Read the model definition and answer for the solid it produces. Units are mm, in the model's axes. A direction names the side the tool comes from. Coordinates: 2 decimals unless noted, no trailing zeros. Write each loop counter-clockwise with the first axis right and the second up, starting at its lowest first coordinate (ties: lowest second). Pieces come first, ordered by that corner, then holes. Notation, with made-up numbers: (-14, -2) -> (26, -2) arc R20 ccw to (26, 16) -> close; hole circle Ø7 at (18.5, 17.5). An arc over 180 degrees is marked (long way). Answer as a JSON object with one key per item and string values. Group by question number.
(1) Which of the six approach directions +Z, -Z, +X, -X, +Y, -Y give full straight-line access (tool end or side, diameter ignored) to faces 1 (the face through (-1.3, -0.6, 3)), 2 (the face through (1.2, -1.2, 0)), 3 (the face through (0, -1.25, 2))?
(2) For a pull along X with two mould halves and no side action, classify faces 4 (the face through (0, 1.25, 2)), 5 (the face through (-0.596, -2.685, 1.479)), 6 (the face through (0, 0, -11.5)) as +X half, -X half, draft (parallel to the pull), parting line (faces both ways), or undercut.
(3) Straight lines are drawn through the part: L1, parallel to Z at x = 0.4, y = 2; L2, parallel to Y at x = 2.45, z = 1.25; L3, parallel to Y at x = -0.9, z = 2. For each, find the intervals that lie inside material, in ascending order.
(4) Find section C-C (z = -0.25). Give the vertices of the cut face in (x, y), then the cut area to 3 significant figures.
(5) Flat-ended cylindrical pins translate along their axes: P1, Ø0.8, axis at x = 0, y = 0, coming from the +Z side; P2, Ø3, axis at x = -1, z = -6.5, coming from the +Y side. Find the tip coordinate at first contact, or state that the pin passes through.
(6) Find section D-D (x = 1.65). Give the vertices of the cut face in (y, z), then the cut area to 3 significant figures.
(7) Find section A-A (y = -0.7). Give the vertices of the cut face in (x, z), then the cut area to 3 significant figures.
(8) Find section B-B (x = 0). Give the vertices of the cut face in (y, z), then the cut area to 4 significant figures.
from build123d import *

# Parameters (mm, degrees)
SKETCH2_R           = 2.75
BOSS_EXTRUDE1_DEPTH = 3
SKETCH3_R           = 1.5
BOSS_EXTRUDE2_DEPTH = 11.5
CUT_EXTRUDE1_DEPTH  = 1.5


with BuildPart() as part:
    # Sketch2 → Boss-Extrude1 (new body)
    with BuildSketch(Plane.XY):
        Circle(SKETCH2_R)
    extrude(amount=BOSS_EXTRUDE1_DEPTH)

    # Sketch3 → Boss-Extrude2 (add)
    with BuildSketch(Plane(origin=(0, 0, 0), x_dir=(-1, 0, 0), z_dir=(0, 0, -1))):
        Circle(SKETCH3_R)
    extrude(amount=BOSS_EXTRUDE2_DEPTH)

    # Sketch4 → Cut-Extrude1 (cut)
    with BuildSketch(Plane.XY.offset(3)):
        Polygon((1.443375673, 0), (0.721687836, 1.25), (-0.721687836, 1.25), (-1.443375673, 0), (-0.721687836, -1.25), (0.721687836, -1.25), align=None)
    extrude(amount=-CUT_EXTRUDE1_DEPTH, mode=Mode.SUBTRACT)


solid = part.part
Results below:
{
 "1": {"face 1": "+Z, +X, -X, +Y, -Y", "face 2": "-Z", "face 3": "+Z"},
 "2": {"face 4": "undercut", "face 5": "parting line", "face 6": "draft"},
 "3": {"L1": "z = 0 to 3", "L2": "y = -1.25 to 1.25", "L3": "y = -2.6 to -0.94, 0.94 to 2.6"},
 "4": {"outline": "circle Ø3 at (0, 0)", "area": "7.07 mm2"},
 "5": {"P1": "stops at z = 1.5", "P2": "stops at y = 1.5"},
 "6": {"outline": "(-2.2, 0) -> (2.2, 0) -> (2.2, 3) -> (-2.2, 3) -> close", "area": "13.2 mm2"},
 "7": {"outline": "(-2.66, 0) -> (-1.33, 0) -> (-1.33, -11.5) -> (1.33, -11.5) -> (1.33, 0) -> (2.66, 0) -> (2.66, 3) -> (1.04, 3) -> (1.04, 1.5) -> (-1.04, 1.5) -> (-1.04, 3) -> (-2.66, 3) -> close", "area": "43.4 mm2"},
 "8": {"outline": "(-2.75, 0) -> (-1.5, 0) -> (-1.5, -11.5) -> (1.5, -11.5) -> (1.5, 0) -> (2.75, 0) -> (2.75, 3) -> (1.25, 3) -> (1.25, 1.5) -> (-1.25, 1.5) -> (-1.25, 3) -> (-2.75, 3) -> close", "area": "47.25 mm2"}
}
